Geometry check sheet. Reference: drawing and pictorial views, mm from the part's lowest x, y, z. A direction names the side the tool comes from. Round coordinates to 2 decimals unless told otherwise and drop trailing zeros. Write each loop counter-clockwise with the first axis right and the second up, starting at its lowest first coordinate (ties: lowest second). Pieces come first, ordered by that corner, then holes. Notation, with made-up numbers: (-22, 80.25) -> (-5, 80.25) arc R38 cw to (-5, 119.25) -> close; hole circle Ø10 at (80.25, 24.25). An arc over 180 degrees is marked (long way). Write item = value, one per line.
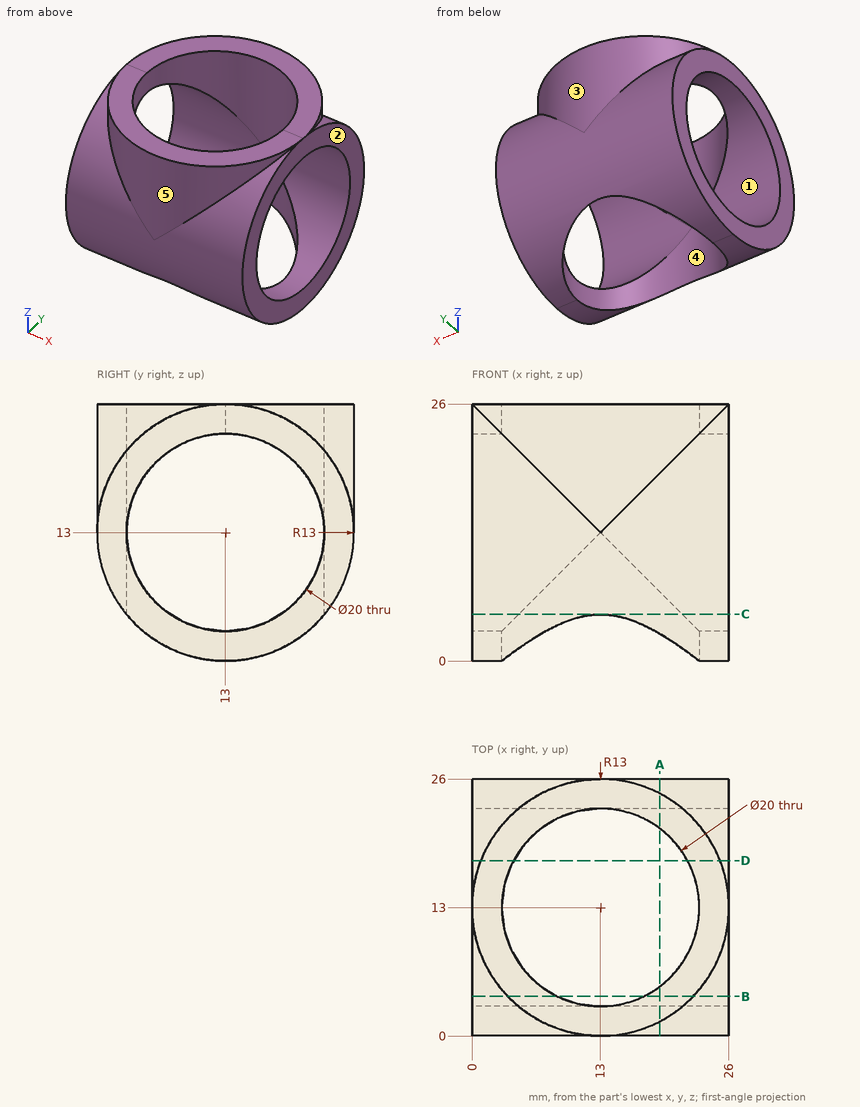
(1) Go/stop test with flat-tipped pins: P1, Ø2, axis at x = 6, y = 3, coming from the -Z side; P2, Ø3, axis at x = 5, z = 7.5, coming from the -Y side; P3, Ø2, axis at x = 3.5, z = 3.5, coming from the +Y side. Record where each tip stops, or that it passes through.
Worked answers:
P1 = 3.62
P2 = 0.63
P3 = 22.84
(2) Sectioned sample at B-B on y = 4. Enter the section's corners in (x, z), then the cut area to 3 significant figures.
Worked answers:
outline = (0, 3.62) -> (8.64, 3.62) -> (8.64, 8.64) -> (0, 8.64) -> close; (0, 17.36) -> (8.64, 17.36) -> (8.64, 26) -> (3.62, 26) -> (3.62, 22.38) -> (0, 22.38) -> close; (17.36, 3.62) -> (26, 3.62) -> (26, 8.64) -> (17.36, 8.64) -> close; (17.36, 17.36) -> (26, 17.36) -> (26, 22.38) -> (22.38, 22.38) -> (22.38, 26) -> (17.36, 26) -> close
area = 210 mm²
(3) Material ranges on L1, parallel to Y at x = 22.75, z = 13; L2, parallel to Y at x = 22.25, z = 1.75; L3, parallel to Z at x = 20.75, y = 6.5, recorded low to high. Write a range as [from, to].
Worked answers:
L1 = [0, 3], [23, 26]
L2 = [6.49, 9.2], [16.8, 19.51]
L3 = [1.74, 5.4], [20.6, 26]
(4) Sectioned sample at D-D on y = 17.75. Enter the section's corners in (x, z).
Worked answers:
outline = (0, 0.9) -> (4.2, 0.9) -> (4.2, 4.2) -> (0, 4.2) -> close; (0, 21.8) -> (4.2, 21.8) -> (4.2, 26) -> (0.9, 26) -> (0.9, 25.1) -> (0, 25.1) -> close; (21.8, 0.9) -> (26, 0.9) -> (26, 4.2) -> (21.8, 4.2) -> close; (21.8, 21.8) -> (26, 21.8) -> (26, 25.1) -> (25.1, 25.1) -> (25.1, 26) -> (21.8, 26) -> close
(5) Sectioned sample at C-C on z = 4.75. Enter the section's corners in (x, y).
Worked answers:
outline = (0, 2.95) -> (26, 2.95) -> (26, 7.35) -> (21.25, 7.35) arc R10 cw to (4.75, 7.35) -> (0, 7.35) -> close; (0, 18.65) -> (4.75, 18.65) arc R10 cw to (21.25, 18.65) -> (26, 18.65) -> (26, 23.05) -> (0, 23.05) -> close
(6) Sectioned sample at A-A on x = 19. Enter the section's corners in (y, z), then the cut area to 3 significant figures.
Worked answers:
outline = (1.47, 19) arc R13 ccw to (5, 2.75) -> (5, 7) arc R10 cw to (5, 19) -> (5, 26) -> (1.47, 26) -> close; (21, 2.75) arc R13 ccw to (24.53, 19) -> (24.53, 26) -> (21, 26) -> (21, 19) arc R10 cw to (21, 7) -> close
area = 142 mm²
(7) Release check for a two-part mould opening along Z. For the marked faces 1 and 2 record: pulls with the +Z half, pulls with the -Z half, needs draft (parallel to the pull), parting line crosses it, or undercut.
Worked answers:
face_1 = undercut
face_2 = needs draft
(8) Access from +Z, -Z, +X, -X, +Y, -Y to the whole of each face (thin tool, end or side, straight path). Record for the marked faces 3, 4 and 5.
Worked answers:
face_3 = +Z, +Y
face_4 = +Z, -Z
face_5 = +Z, -Y
